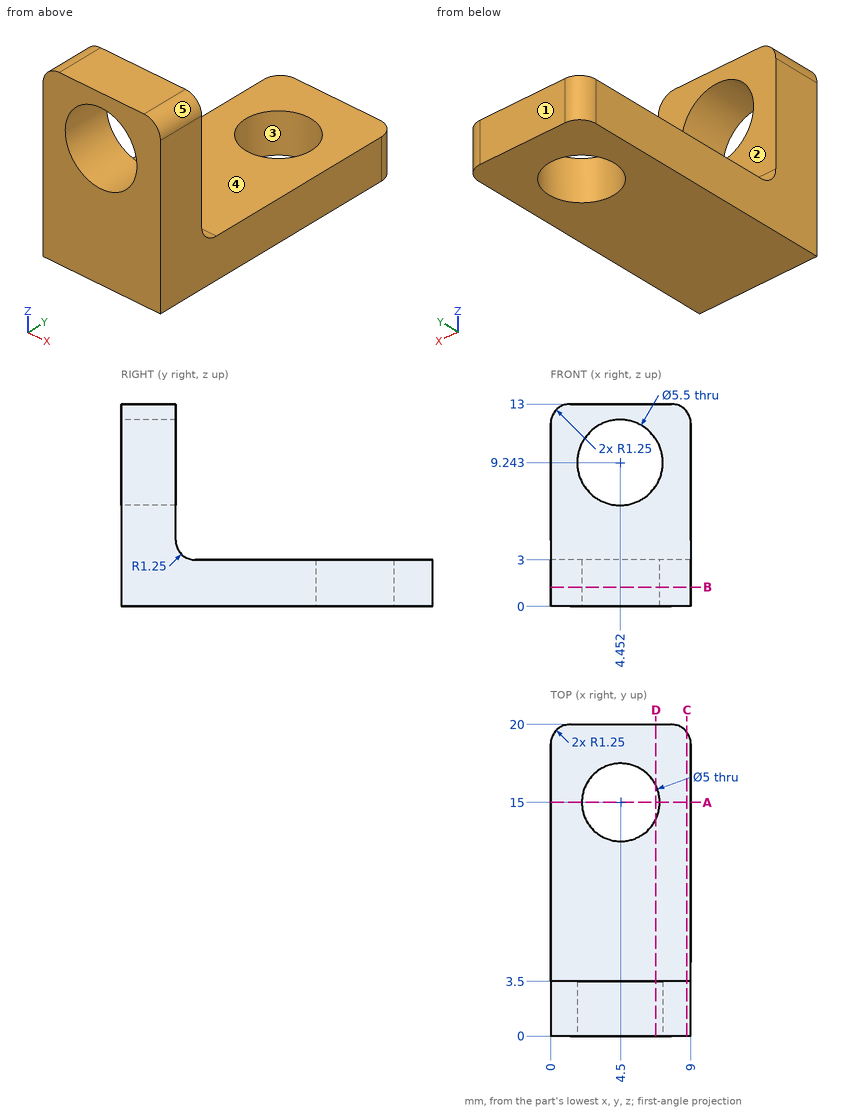
Geometry: see drawing. Coordinates: mm, zero at the bounding-box minimum. A direction names the side the tool comes from. Coordinates: 2 decimals unless noted, no trailing zeros. Loops run counter-clockwise (first coordinate to the right, second up) from the corner with the lowest first, then second, coordinate; pieces in that order, holes last. Notation, with made-up numbers: M -23,81 L -14,81 A16 cw -14,104 Z; hole C 2,53.5 d3. An arc over 180 degrees is marked long. Put each result on its own line as item: value. Start each with the question number.
1) Cut plane B-B on z = 1.25. Return the cut outline in (x, y), then the cut area to 3 significant figures.
2) Cut plane A-A on y = 15. Return the cut outline in (x, z).
3) Ray query, L1, parallel to Y at x = 4.5, z = 1.55; L2, parallel to Z at x = 2, y = 11.75; L3, parallel to Y at x = 5.25, z = 6.5. Return the intervals inside material, ascending. Write a range as from..to.
4) Contact query for flat-ended pins moving along their axis: pin 1 Ø2 at (x, z) = (7.5, 9.5) entering from +Y; pin 2 Ø4.5 at (x, y) = (4, 13.5) entering from +Z. Output: stop coordinate, or through.
5) Pull-direction query (X, two-part tool) for the marked faces 3, 4 and 5; classes: pulls with the +X half, pulls with the -X half, needs draft (parallel to the pull), parting line crosses it, or undercut.
6) Cut plane D-D on x = 6.75. Return the cut outline in (y, z).
7) Reachability of the marked faces 1 and 2 from +Z, -Z, +X, -X, +Y, -Y: full face, straight path, thin tool, end or side. Return the list, or none.
8) Cut plane C-C on x = 8.75. Return the cut outline in (y, z).
The answers:
1. outline: M 0,0 L 9,0 L 9,18.75 A1.25 ccw 7.75,20 L 1.25,20 A1.25 ccw 0,18.75 Z; hole C 4.5,15 d5
1. area: 160 mm²
2. outline: M 0,0 L 2,0 L 2,3 L 0,3 Z; M 7,0 L 9,0 L 9,3 L 7,3 Z
3. L1: y = 0..12.5, 17.5..20
3. L2: z = 0..3
3. L3: y = 0..3.5
4. pin 1: stops at y = 3.5
4. pin 2: stops at z = 3
5. face 3: undercut
5. face 4: needs draft
5. face 5: pulls with the +X half
6. outline: M 0,0 L 13.91,0 L 13.91,3 L 4.75,3 A1.25 cw 3.5,4.25 L 3.5,7.73 L 0,7.73 Z; M 0,10.75 L 3.5,10.75 L 3.5,13 L 0,13 Z; M 16.09,0 L 20,0 L 20,3 L 16.09,3 Z
7. face 1: +Z, -Z, +X, -X, +Y
7. face 2: +Z, +X, -X, +Y
8. outline: M 0,0 L 19.5,0 L 19.5,3 L 4.75,3 A1.25 cw 3.5,4.25 L 3.5,12.5 L 0,12.5 Z
